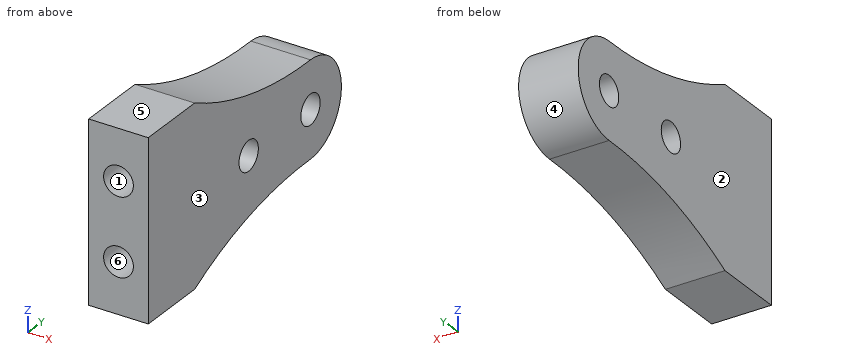
```python
from build123d import *

# Parameters (mm, degrees)
BOSS_EXTRUDE1_DEPTH         = 2.5
TAP_DRILL_FOR_M3_TAP1_D     = 2.5
TAP_DRILL_FOR_M3_TAP2_D     = 2.5
TAP_DRILL_FOR_M3_TAP2_DEPTH = 5
TAP_DRILL_FOR_M3_TAP2_TIP   = 0.751075774


with BuildPart() as part:
    # Sketch1 → Boss-Extrude1 (new, symmetric)
    with BuildSketch(Plane(origin=(0, 0, 0), x_dir=(0, 0, -1), z_dir=(1, 0, 0))):
        with BuildLine():
            Line((-7.5, -12.5), (7.5, -12.5))
            Line((7.5, -12.5), (7.5, -6.5))
            ThreePointArc((7.5, -6.5), (4.834023326, 0.786272109), (4, 8.5))
            ThreePointArc((4, 8.5), (0, 12.5), (-4, 8.5))
            ThreePointArc((-4, 8.5), (-4.834023326, 0.786272109), (-7.5, -6.5))
            Line((-7.5, -6.5), (-7.5, -12.5))
        make_face()
    extrude(amount=BOSS_EXTRUDE1_DEPTH, both=True)

    # Tap Drill for M3 Tap1 (through all)
    with Locations(Plane(origin=(2.5, 0, 0), x_dir=(0, 0, -1), z_dir=(1, 0, 0))):
        with Locations((0, 8.5), (0, 0.5)):
            Hole(TAP_DRILL_FOR_M3_TAP1_D / 2)

    # Tap Drill for M3 Tap2
    with Locations(Plane(origin=(0, -12.5, 0), x_dir=(-1, 0, 0), z_dir=(0, -1, 0))):
        with Locations((0, -3.25), (0, 3.25)):
            Hole(TAP_DRILL_FOR_M3_TAP2_D / 2, depth=TAP_DRILL_FOR_M3_TAP2_DEPTH)
            with Locations((0, 0, -(TAP_DRILL_FOR_M3_TAP2_DEPTH + TAP_DRILL_FOR_M3_TAP2_TIP / 2))):  # 118° drill point
                Cone(0, TAP_DRILL_FOR_M3_TAP2_D / 2, TAP_DRILL_FOR_M3_TAP2_TIP, mode=Mode.SUBTRACT)


solid = part.part
```
CAD build for the part. Positions are in the model's coordinates, mm. Face numbers are marked on the shaded views. A direction names the side the tool comes from. Give positions to 0.01 mm unless a question says otherwise; leave off trailing zeros. Order: outer loops, then holes, each group sorted by start corner. A loop starts at its lowest first (then second) coordinate and runs counter-clockwise, first axis right, second up.
(1) Tool access for the marked faces 5 and 6: list every direction of +Z, -Z, +X, -X, +Y, -Y with a clear straight run to the whole face (end or side of a thin tool).
(2) Saw through at A-A, the plane z = 0. Give the cut face in (x, y).
(3) Saw through at C-C, the plane x = -1.85. Give the cut face in (y, z), then the cut area to 3 significant figures.
(4) Flat gauge pins, fed straight in: pin 1 (2 mm diameter, centred on y = 0.5, z = 0, fed in from -X); pin 2 (3 mm diameter, centred on x = 0, z = -3.25, fed in from -Y); pin 3 (1.5 mm diameter, centred on x = 0, y = 6, fed in from -Z). Where does each tip first touch, or does it go through?
(5) Saw through at D-D, the plane y = -10.25. Give the cut face in (x, z).
(6) Drill centre lines: L1, parallel to Y at x = -0.95, z = 0; L2, parallel to Z at x = 0, y = -9.9; L3, parallel to Y at x = -2.1, z = 1. Where is each one in solid material? Low to high.
(7) Mould opens along X. For the marked faces 1, 2, 3 and 4 say: released by +X, released by -X, zero draft, split by the parting line, or undercut.
(8) Saw through at B-B, the plane y = 0.5. Give the cut face in (x, z), then the cut area to 3 significant figures.
Results found:
1. face 5: +Z, +X, -X, +Y, -Y
1. face 6: -Y
2. outline: (-2.5, -12.5) - (2.5, -12.5) - (2.5, -0.75) - (-2.5, -0.75) - close; (-2.5, 1.75) - (2.5, 1.75) - (2.5, 7.25) - (-2.5, 7.25) - close; (-2.5, 9.75) - (2.5, 9.75) - (2.5, 12.5) - (-2.5, 12.5) - close
3. outline: (-12.5, -7.5) - (-6.5, -7.5) arc R32 cw to (8.5, -4) arc R4 ccw to (8.5, 4) arc R32 cw to (-6.5, 7.5) - (-12.5, 7.5) - close; hole circle Ø2.5 at (0.5, 0); hole circle Ø2.5 at (8.5, 0)
3. area: 258 mm2
4. pin 1: passes through
4. pin 2: stops at y = -12.5
4. pin 3: stops at z = -4.12
5. outline: (-2.5, -7.5) - (2.5, -7.5) - (2.5, 7.5) - (-2.5, 7.5) - close; hole circle Ø2.5 at (0, -3.25); hole circle Ø2.5 at (0, 3.25)
6. L1: y = -12.5 to -0.75, 1.75 to 7.25, 9.75 to 12.5
6. L2: z = -7.5 to -4.5, -2 to 2, 4.5 to 7.5
6. L3: y = -12.5 to -0.25, 1.25 to 7.75, 9.25 to 12.37
7. face 1: undercut
7. face 2: released by -X
7. face 3: released by +X
7. face 4: zero draft
8. outline: (-2.5, -4.9) - (2.5, -4.9) - (2.5, -1.25) - (-2.5, -1.25) - close; (-2.5, 1.25) - (2.5, 1.25) - (2.5, 4.9) - (-2.5, 4.9) - close
8. area: 36.5 mm2
